Verification items for the finished model (mm, model axes). A direction names the side the tool comes from. Round coordinates to 2 decimals unless told otherwise and drop trailing zeros. Write each loop counter-clockwise with the first axis right and the second up, starting at its lowest first coordinate (ties: lowest second). Pieces come first, ordered by that corner, then holes. Notation, with made-up numbers: (-27, -6.5) -> (1, -6.5) arc R20 ccw to (1, 19.5) -> close; hole circle Ø7 at (-25, -2). An arc over 180 degrees is marked (long way). Answer as a JSON object with one key per item and string values. Group by question number.
(1) Sectioned sample at A-A on x = -134. Record the cut outline in (y, z).
(2) Scan lines: L1, parallel to X at y = 3, z = 18; L2, parallel to Z at x = -172, y = 1.95. Record each from-to range of solid material in increasing order. Write a range as from..to.
(3) Sectioned sample at B-B on z = 72. Record the cut outline in (x, y).
(4) Set-up check for faces 1 (the face through (-159.018, 2, -3)), 2 (the face through (-189.018, 2, 45)), 3 (the face through (-94, 2, 90)), 4 (the face through (-187, 2, 40)): record each of +Z, -Z, +X, -X, +Y, -Y from which the full face is reachable in a straight line by a thin tool's end or side.
(5) Draft check along Z on faces 5 (the face through (-144, 2, -5)), 6 (the face through (-186, 2, 30)), 7 (the face through (-4.018, 2, 92)). Enter one of: released by +Z, released by -Z, zero draft, split by the parting line, or undercut.
(6) Gauge pin test, flat ends, axial feed: pin 1 Ø2.5 at (y, z) = (3, 92) entering from -X; pin 2 Ø1.5 at (x, y) = (-186, 1.5) entering from +Z; pin 3 Ø1 at (y, z) = (1, 56.5) entering from +X. Record the tip position at first contact, or that the pin passes through.
```python
from build123d import *

# Parameters (mm, degrees)
BOSS_EXTRUDE3_DEPTH = 5


with BuildPart() as part:
    # Sketch2 → Boss-Extrude3 (new body)
    with BuildSketch(Plane(origin=(0, 0, 0), x_dir=(1, 0, 0), z_dir=(0, 1, 0))):
        Polygon((-4.018396485, -10), (-4.018396485, -20), (0.981603515, -20), (0.981603515, -30), (-4.018396485, -30), (-4.018396485, -40), (0.981603515, -40), (0.981603515, -50), (-4.018396485, -50), (-4.018396485, -60), (0.981603515, -60), (0.981603515, -70), (-4.018396485, -70), (-4.018396485, -80), (0.981603515, -80), (0.981603515, -90), (-4.018396485, -90), (-4.018396485, -95), (-9.018396485, -95), (-9.018396485, -90), (-19.018396485, -90), (-19.018396485, -95), (-29.018396485, -95), (-29.018396485, -90), (-39.018396485, -90), (-39.018396485, -95), (-49.018396485, -95), (-49.018396485, -90), (-59.018396485, -90), (-59.018396485, -95), (-69.018396485, -95), (-69.018396485, -90), (-79.018396485, -90), (-79.018396485, -95), (-89.018396485, -95), (-89.018396485, -90), (-99.018396485, -90), (-99.018396485, -95), (-109.018396485, -95), (-109.018396485, -90), (-119.018396485, -90), (-119.018396485, -95), (-129.018396485, -95), (-129.018396485, -90), (-139.018396485, -90), (-139.018396485, -95), (-149.018396485, -95), (-149.018396485, -90), (-159.018396485, -90), (-159.018396485, -95), (-169.018396485, -95), (-169.018396485, -90), (-179.018396485, -90), (-179.018396485, -95), (-184.018396485, -95), (-184.018396485, -90), (-189.018396485, -90), (-189.018396485, -80), (-184.018396485, -80), (-184.018396485, -70), (-189.018396485, -70), (-189.018396485, -60), (-184.018396485, -60), (-184.018396485, -50), (-189.018396485, -50), (-189.018396485, -40), (-184.018396485, -40), (-184.018396485, -30), (-189.018396485, -30), (-189.018396485, -20), (-184.018396485, -20), (-184.018396485, -10), (-189.018396485, -10), (-189.018396485, 0), (-184.018396485, 0), (-184.018396485, 5), (-179.018396485, 5), (-179.018396485, 0), (-169.018396485, 0), (-169.018396485, 5), (-159.018396485, 5), (-159.018396485, 0), (-149.018396485, 0), (-149.018396485, 5), (-139.018396485, 5), (-139.018396485, 0), (-129.018396485, 0), (-129.018396485, 5), (-119.018396485, 5), (-119.018396485, 0), (-109.018396485, 0), (-109.018396485, 5), (-99.018396485, 5), (-99.018396485, 0), (-89.018396485, 0), (-89.018396485, 5), (-79.018396485, 5), (-79.018396485, 0), (-69.018396485, 0), (-69.018396485, 5), (-59.018396485, 5), (-59.018396485, 0), (-49.018396485, 0), (-49.018396485, 5), (-39.018396485, 5), (-39.018396485, 0), (-29.018396485, 0), (-29.018396485, 5), (-19.018396485, 5), (-19.018396485, 0), (-9.018396485, 0), (-9.018396485, 5), (-4.018396485, 5), (-4.018396485, 0), (0.981603515, 0), (0.981603515, -10), align=None)
    extrude(amount=BOSS_EXTRUDE3_DEPTH)


solid = part.part
```
Computed values:
{
 "1": {"outline": "(0, 0) -> (5, 0) -> (5, 90) -> (0, 90) -> close"},
 "2": {"L1": "-184.02..-4.02", "L2": "0..90"},
 "3": {"outline": "(-184.02, 0) -> (-4.02, 0) -> (-4.02, 5) -> (-184.02, 5) -> close"},
 "4": {"face 1": "-Z, +Y, -Y", "face 2": "+Z, -Z, -X, +Y, -Y", "face 3": "+Z, +Y, -Y", "face 4": "-X, +Y, -Y"},
 "5": {"face 5": "released by -Z", "face 6": "undercut", "face 7": "zero draft"},
 "6": {"pin 1": "x = -184.02", "pin 2": "z = 90", "pin 3": "x = -4.02"}
}
